```python
from build123d import *

# Parameters (mm, degrees)
SKETCH1_R           = 1.55
SKETCH1_R_2         = 2.05
BOSS_EXTRUDE1_DEPTH = 4
SKETCH2_R           = 2
BOSS_EXTRUDE2_DEPTH = 4
SKETCH3_W           = 20
SKETCH3_H           = 4
BOSS_EXTRUDE3_DEPTH = 36.5
SKETCH4_R           = 1.55
CUT_EXTRUDE1_DEPTH  = 5
CUT_EXTRUDE2_DEPTH  = 2
BOSS_EXTRUDE4_DEPTH = 4
FILLET1_R           = 2
FILLET2_R           = 3
SKETCH7_W           = 8
SKETCH7_H           = 26
CUT_EXTRUDE3_DEPTH  = 10
FILLET3_R           = 2
SKETCH8_R           = 2.85
CUT_EXTRUDE4_DEPTH  = 2


with BuildPart() as part:
    # Sketch1 → Boss-Extrude1 (new body)
    with BuildSketch(Plane.XY):
        with BuildLine():
            Line((-25, -35.5), (0, -35.5))
            Line((0, -35.5), (7.872983346, -35.5))
            Line((7.872983346, -35.5), (7.872983346, -26.5))
            ThreePointArc((7.872983346, -26.5), (4.377000516, -22.531881215), (0, -25.5))
            Line((0, -25.5), (-25, -25.5))
            Line((-25, -25.5), (-25, -35.5))
        make_face()
        with Locations((-20, -30.5)):
            Circle(SKETCH1_R, mode=Mode.SUBTRACT)
        with Locations((-5, -30.5)):
            Circle(SKETCH1_R, mode=Mode.SUBTRACT)
        with Locations((3.872983346, -26.5)):
            Circle(SKETCH1_R_2, mode=Mode.SUBTRACT)
    extrude(amount=BOSS_EXTRUDE1_DEPTH)

    # Sketch2 → Boss-Extrude2 (add)
    with BuildSketch(Plane.XY.offset(4)):
        with BuildLine():
            Line((7.872983346, -35.5), (7.872983346, -26.5))
            ThreePointArc((7.872983346, -26.5), (7.513600322, -24.842921839), (6.50002933, -23.483606557))
            Line((6.50002933, -23.483606557), (49.483635887, -60.919011822))
            ThreePointArc((49.483635887, -60.919011822), (49.872983346, -66.562451248), (44.22954392, -66.951798707))
            Line((44.22954392, -66.951798707), (8.116358245, -35.5))
            Line((8.116358245, -35.5), (7.872983346, -35.5))
        make_face()
        with Locations((46.856589904, -63.935405265)):
            Circle(SKETCH2_R, mode=Mode.SUBTRACT)
    extrude(amount=-BOSS_EXTRUDE2_DEPTH)

    # Sketch3 → Boss-Extrude3 (add)
    with BuildSketch(Plane.XZ.offset(35.5)):
        with Locations((-15, 2)):
            Rectangle(SKETCH3_W, SKETCH3_H)
    extrude(amount=BOSS_EXTRUDE3_DEPTH)

    # Sketch4 → Cut-Extrude1 (cut, through all)
    with BuildSketch(Plane.XY.offset(4)):
        with Locations((-20, -67)):
            Circle(SKETCH4_R)
        with Locations((-10, -67)):
            Circle(SKETCH4_R)
    extrude(amount=-CUT_EXTRUDE1_DEPTH, mode=Mode.SUBTRACT)

    # Sketch5 → Cut-Extrude2 (cut)
    with BuildSketch(Plane(origin=(0, 0, 0), x_dir=(-1, 0, 0), z_dir=(0, 0, -1))):
        Polygon((22.85, -68.645448267), (22.85, -65.354551733), (20, -63.709103466), (17.15, -65.354551733), (17.15, -68.645448267), (20, -70.290896534), align=None)
        Polygon((12.85, -68.645448267), (12.85, -65.354551733), (10, -63.709103466), (7.15, -65.354551733), (7.15, -68.645448267), (10, -70.290896534), align=None)
    extrude(amount=-CUT_EXTRUDE2_DEPTH, mode=Mode.SUBTRACT)

    # Sketch6 → Boss-Extrude4 (add)
    with BuildSketch(Plane(origin=(0, 0, 0), x_dir=(-1, 0, 0), z_dir=(0, 0, -1))):
        with BuildLine():
            ThreePointArc((-44.22954392, -66.951798707), (-45.454016157, -67.681441421), (-46.856589904, -67.935405265))
            Line((-46.856589904, -67.935405265), (5, -67.935405265))
            Line((5, -67.935405265), (5, -62.935405265))
            Line((5, -62.935405265), (-39.617891547, -62.935405265))
            Line((-39.617891547, -62.935405265), (-44.22954392, -66.951798707))
        make_face()
    extrude(amount=-BOSS_EXTRUDE4_DEPTH)

    # Fillet1
    fillet1_edges = [part.edges().sort_by_distance(p)[0] for p in [
        (39.617891547, -62.935405265, 2),
        (-5, -62.935405265, 2),
        (8.116358245, -35.5, 2),
        (-5, -35.5, 2),
    ]]
    fillet(fillet1_edges, radius=FILLET1_R)

    # Fillet2
    fillet2_edges = [part.edges().sort_by_distance(p)[0] for p in [
        (-25, -25.5, 2),
        (-5, -72, 2),
        (-25, -72, 2),
    ]]
    fillet(fillet2_edges, radius=FILLET2_R)

    # Sketch7 → Cut-Extrude3 (cut)
    with BuildSketch(Plane(origin=(0, 0, 0), x_dir=(-1, 0, 0), z_dir=(0, 0, -1))):
        with Locations((15, -48.75)):
            Rectangle(SKETCH7_W, SKETCH7_H)
    extrude(amount=-CUT_EXTRUDE3_DEPTH, mode=Mode.SUBTRACT)

    # Fillet3
    fillet3_edges = [part.edges().sort_by_distance(p)[0] for p in [
        (-11, -61.75, 2),
        (-11, -35.75, 2),
        (-19, -35.75, 2),
        (-19, -61.75, 2),
    ]]
    fillet(fillet3_edges, radius=FILLET3_R)

    # Sketch8 → Cut-Extrude4 (cut)
    with BuildSketch(Plane.XY.offset(4)):
        with Locations((-20, -30.5)):
            Circle(SKETCH8_R)
        with Locations((-5, -30.5)):
            Circle(SKETCH8_R)
    extrude(amount=-CUT_EXTRUDE4_DEPTH, mode=Mode.SUBTRACT)


solid = part.part
```
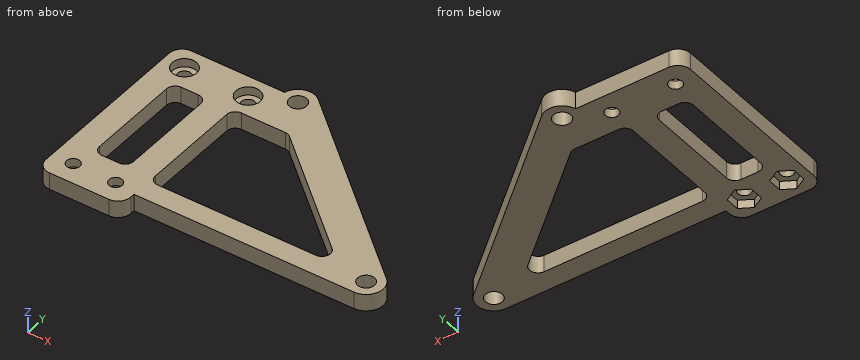
Read the model definition and answer for the solid it produces. Units are mm, in the model's axes. Give positions to 0.01 mm unless a question says otherwise; leave off trailing zeros. Write each loop counter-clockwise with the first axis right and the second up, starting at its lowest first coordinate (ties: lowest second). Pieces come first, ordered by that corner, then holes. Notation, with made-up numbers: M 75.5,61.5 L 99.5,61.5 A37 ccw 99.5,100.5 Z; hole C -13,-12 d9. An arc over 180 degrees is marked long. Put each result on its own line as item: value. Start each with the question number.
1. The part is cut by section B-B, the plane y = -26.5. Give the vertices of the cut face in (x, z), and give its area (3 significant figures).
2. Each of these flat-tipped pins is pushed along its axis until it touches: pin 1 Ø4.5 at (x, y) = (46.86, -63.94) entering from +Z; pin 2 Ø1.2 at (x, z) = (24.5, 1) entering from +Y; pin 3 Ø2 at (x, z) = (3.5, 2) entering from -Y; pin 4 Ø4.5 at (x, y) = (-20, -66.5) entering from -Z. Where does it stop, or does it pass through?
3. The part is cut by section D-D, the plane x = 41. Give the vertices of the cut face in (y, z), and give its area (3 significant figures).
4. The part is cut by section C-C, the plane y = -45.5. Give the vertices of the cut face in (x, z).
5. The part is cut by section A-A, the plane x = -1. Give the vertices of the cut face in (y, z), and give its area (3 significant figures).
6. Consider line 1 along Y through (x, z) = (-18, 0.9); line 2 along X through (y, z) = (-30.5, 1); line 3 along Y through (x, z) = (-13, 0.65). Determine where each line is inside the solid, lowest interval first.
Final values:
1. outline: M -24.24,0 L 1.82,0 L 1.82,4 L -24.24,4 Z; M 5.92,0 L 9.96,0 L 9.96,4 L 5.92,4 Z
1. area: 120 mm²
2. pin 1: stops at z = 4
2. pin 2: stops at y = -38.64
2. pin 3: stops at y = -67.94
2. pin 4: stops at z = 2
3. outline: M -67.94,0 L -53.53,0 L -53.53,4 L -67.94,4 Z
3. area: 57.6 mm²
4. outline: M -25,0 L -19,0 L -19,4 L -25,4 Z; M -11,0 L -5,0 L -5,4 L -11,4 Z; M 19.6,0 L 31.78,0 L 31.78,4 L 19.6,4 Z
5. outline: M -67.94,0 L -62.94,0 L -62.94,4 L -67.94,4 Z; M -35.5,0 L -25.5,0 L -25.5,4 L -35.5,4 Z
5. area: 60.0 mm²
6. line 1: y = -72 to -69.14, -64.86 to -61.48, -36.02 to -25.5
6. line 2: x = -25 to -21.55, -18.45 to -6.55, -3.45 to 14.56
6. line 3: y = -72 to -61.75, -35.75 to -25.5
